Here's the drawing with two shaded views (mm, measured from the low corner). I have some questions. A direction names the side the tool comes from. Round coordinates to 2 decimals unless told otherwise and drop trailing zeros. Write each loop counter-clockwise with the first axis right and the second up, starting at its lowest first coordinate (ties: lowest second). Pieces come first, ordered by that corner, then holes. Notation, with made-up numbers: M 23.5,54 L 81.5,54 A12 cw 81.5,60 Z; hole C 40,78.5 d8. An arc over 180 degrees is marked long. Answer as a JSON object with one key per item and string values. Group by question number.
1) Suppose I cut it at D-D, the plane x = 11.75. Write out the boundary of the cut face in (y, z), and give its area (3 significant figures).
2) Suppose I cut it at A-A, the plane z = 4.5. Write out the boundary of the cut face in (x, y), and give its area (3 significant figures).
3) If we mould it in two halves opening along X, with no side actions, what happens to the marked faces 3, 4 and 5? For each: +X half, -X half, draft (parallel to the pull), parting line (faces both ways), or undercut.
4) Please list where these lines run through material, in increasing order: L1, parallel to X at y = 4.5, z = 4.5; L2, parallel to X at y = 2.25, z = 4.5; L3, parallel to X at y = 6, z = 7. Write a range as [from, to].
5) On a 3-axis mill with a long thin cutter (end or side, diameter ignored), from which of +Z, -Z, +X, -X, +Y, -Y can I reach the whole of each face in a straight line? I mean the marked faces 1 and 2. Say none if no direction works.
6) I'm going to push a flat-ended pin straight in: pin 1 Ø1 at (x, z) = (10.5, 1.5) entering from +Y. Where does the tip first touch, or does it pass through?
7) Suppose I cut it at C-C, the plane y = 2.5. Write out the boundary of the cut face in (x, z).
8) Suppose I cut it at B-B, the plane x = 18.8. Write out the boundary of the cut face in (y, z).
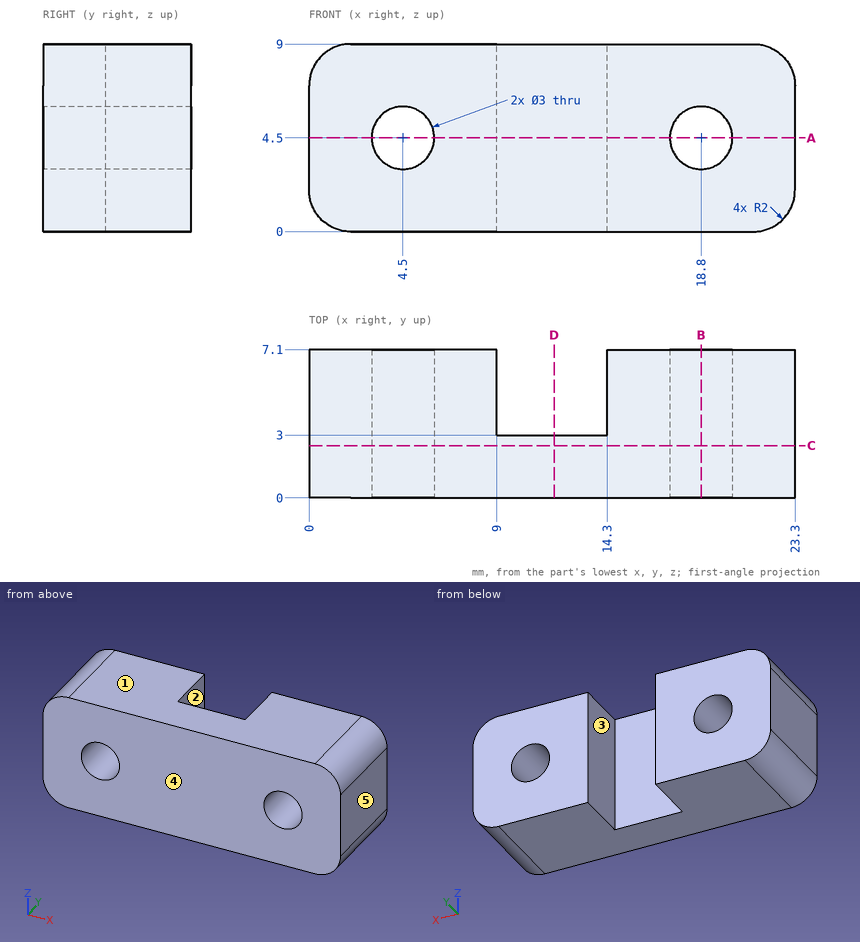
Results:
{
 "1": {"outline": "M 0,0 L 3,0 L 3,9 L 0,9 Z", "area": "27.0 mm^2"},
 "2": {"outline": "M 0,0 L 3,0 L 3,7.1 L 0,7.1 Z; M 6,0 L 17.3,0 L 17.3,7.1 L 14.3,7.1 L 14.3,3 L 9,3 L 9,7.1 L 6,7.1 Z; M 20.3,0 L 23.3,0 L 23.3,7.1 L 20.3,7.1 Z", "area": "101 mm^2"},
 "3": {"face 3": "undercut", "face 4": "draft", "face 5": "+X half"},
 "4": {"L1": "[0, 3], [6, 9], [14.3, 17.3], [20.3, 23.3]", "L2": "[0, 3], [6, 17.3], [20.3, 23.3]", "L3": "[0, 9], [14.3, 23.3]"},
 "5": {"face 1": "+Z, +X, -X, +Y, -Y", "face 2": "+Z, -Z, +Y"},
 "6": {"pin 1": "y = 3"},
 "7": {"outline": "M 0,2 A2 ccw 2,0 L 21.3,0 A2 ccw 23.3,2 L 23.3,7 A2 ccw 21.3,9 L 2,9 A2 ccw 0,7 Z; hole C 4.5,4.5 d3; hole C 18.8,4.5 d3"},
 "8": {"outline": "M 0,0 L 7.1,0 L 7.1,3 L 0,3 Z; M 0,6 L 7.1,6 L 7.1,9 L 0,9 Z"}
}
